Can you work these out from the model? Positions are in its coordinate system, mm. Face numbers are marked on the shaded views. A direction names the side the tool comes from. Give positions to 0.01 mm unless a question says otherwise; leave off trailing zeros. Order: outer loops, then holes, each group sorted by start corner. A loop starts at its lowest first (then second) coordinate and runs counter-clockwise, first axis right, second up. Notation, with made-up numbers: M -36.5,-12.75 L 1.5,-12.75 A23 cw 1.5,13.25 Z; hole C -3.5,86.5 d5. An arc over 180 degrees is marked long. One line per question, with ' | ' between items. Start each with the question number.
1) I'm going to push flat-ended pins straight in: pin 1 Ø2.5 at (x, z) = (255.5, 19) entering from +Y; pin 2 Ø6.5 at (x, y) = (270, -10) entering from +Z; pin 3 Ø3 at (x, y) = (206.5, -0.5) entering from +Z. Where does each tip first touch, or does it pass through?
2) For the marked faces 4 and 5, which set-ups out of +Z, -Z, +X, -X, +Y, -Y let a thin tool reach every point of the face, with its end or its side?
3) If we section it at D-D, the plane z = 14: Please give me the cut outline in (x, y).
4) If we section it at A-A, the plane z = 49: Please give me the cut outline in (x, y), plus the area to 3 significant figures.
5) Please list where these lines run through material, in increasing order: line 1 along Y through (x, z) = (10, 2.5); line 2 along X through (y, z) = (4, 20); line 3 along X through (y, z) = (17.05, 20). Write a range as [from, to].
6) Thinking about a two-plate mould opening in X: for the marked faces 1, 2 and 3, which applies, +X half, -X half, draft (parallel to the pull), parting line (faces both ways), or undercut?
7) If we section it at C-C, the plane x = 98.5: Please give me the cut outline in (y, z).
8) If we section it at B-B, the plane y = 3: Please give me the cut outline in (x, z), plus the area to 3 significant figures.
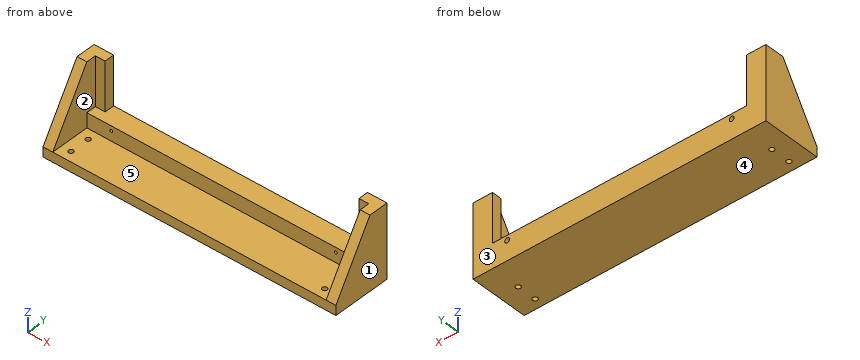
Autodesk Inventor part; units mm, degrees
ref_plane "작업 평면1" through (140, -40, 0) normal (1, 0, 0) x (0, 0, -1)
ref_plane "YZ Plane" through (0, 0, 0) normal (1, 0, 0) x (0, 1, 0)
ref_plane "XZ Plane" through (0, 0, 0) normal (0, 1, 0) x (-1, 0, 0)
sketch "스케치1" plane through (0, 0, 0) normal (0, 0, 1) x (1, 0, 0)
  line L0 (0, 10) -> (0, 0)
  line L1 (-10, 10) -> (-10, 20)
  line L2 (-10, 20) -> (290, 20)
  line L3 (290, 20) -> (290, 10)
  line L4 (0, 0) -> (280, 0)
  line L5 (290, 10) -> (290, -40)
  line L6 (-10, 10) -> (-10, -40)
  line L7 (-10, -40) -> (290, -40)
  line L8 (0, 10) -> (10, 10)
  line L9 (10, 10) -> (10, 20)
  line L10 (140, 20) -> (140, 10)
  line L11 (0, 0) -> (-10, 0)
  line L12 (280, 10) -> (280, 0)
  line L13 (280, 10) -> (270, 10)
  line L14 (270, 10) -> (270, 20)
  line L15 (280, 0) -> (290, 0)
  point P0 (140, 0)
  dimension "d2" = 10
  dimension "d5" = 10
  dimension "d6" = 300
  dimension "d9" = 60
  dimension "d12" = 10
  dimension "d13" = 10
extrude "돌출1" add sketch "스케치1" along normal blind 25 contours L8 L9 L2 L14 L13 L12 L4 L0 | L0 L11 L6 L1 L2 L9 L8 | L12 L13 L14 L2 L3 L5 L15
extrude "돌출2" add sketch "스케치1" along normal blind 10 contours L8 L9 L2 L14 L13 L12 L4 L0 | L4 L15 L5 L7 L6 L11
extrude "돌출3" add sketch "스케치1" along normal blind 75 contours L0 L11 L6 L1 L2 L9 L8 | L12 L13 L14 L2 L3 L5 L15
sketch "스케치2" plane through (-10, -40, 0) normal (-1, 0, 0) x (0, 0, 1)
  line L0 (0, 60) -> (0, 0)
  line L1 (0, 0) -> (10, 0)
  line L2 (10, 40) -> (10, 0)
  line L3 (10, 40) -> (75, 40)
  line L4 (75, 60) -> (75, 40)
  line L5 (0, 60) -> (75, 60)
  line L6 (75, 40) -> (10, 0)
  point P0 (0, 40)
extrude "돌출4" add sketch "스케치2" against normal up to surface (10 mm away) contours L2 L3 L6
ref_plane "작업 평면1" through (140, -40, 0) normal (1, 0, 0) x (0, 0, -1)
mirror "미러1" about plane through (140, -40, 0) normal (1, 0, 0) of "돌출4"
sketch "스케치3" plane through (0, 0, 10) normal (0, 0, 1) x (1, 0, 0)
  circle A0 centre (10, -10) radius 2.5
  circle A1 centre (270, -10) radius 2.5
  line L0 (270, 20) -> (10, 20)
  line L1 (290, -40) -> (290, 0)
  line L2 (-10, -40) -> (-10, 0)
  circle A2 centre (10, -30) radius 2.5
  circle A3 centre (270, -30) radius 2.5
  point P0 (0, 0)
  dimension "d18" = 30
  dimension "d19" = 5
  dimension "d20" = 20
  dimension "d21" = 20
  dimension "d24" = 5
  dimension "d25" = 20
extrude "돌출5" cut sketch "스케치3" against normal through all
sketch "스케치4" plane through (-10, 20, 0) normal (0, 1, 0) x (1, 0, 0)
  line L0 (280, -25) -> (280, -75)
  line L1 (20, -25) -> (20, -75)
  line L2 (280, -25) -> (20, -25)
  point P0 (10, 0)
  point P1 (35, -20)
  point P2 (265, -20)
  dimension "d26" = 15
  dimension "d27" = 15
  dimension "d28" = 5
hole "구멍1" at (25, 20, 20) at (255, 20, 20) direction (0, -1, 0) diameter 3 end through all counterbore diameter 5 counterbore depth 5
properties part number "ModuleConnector"
Results found:
1) pin 1: stops at y = 15 | pin 2: stops at z = 10 | pin 3: stops at z = 25
2) face 4: -Z, +X, -X, +Y, -Y | face 5: +Z, -Y
3) outline: M -10,-37.54 L 0,-37.54 L 0,0 L 280,0 L 280,-37.54 L 290,-37.54 L 290,20 L -10,20 Z
4) outline: M -10,-16 L 0,-16 L 0,10 L 10,10 L 10,20 L -10,20 Z; M 270,10 L 280,10 L 280,-16 L 290,-16 L 290,20 L 270,20 Z | area: 920 mm²
5) line 1: y = [-40, -32.5], [-27.5, -12.5], [-7.5, 20] | line 2: x = [-10, 23.5], [26.5, 253.5], [256.5, 290] | line 3: x = [-10, 22.5], [27.5, 252.5], [257.5, 290]
6) face 1: +X half | face 2: undercut | face 3: draft
7) outline: M -40,0 L 20,0 L 20,25 L 0,25 L 0,10 L -40,10 Z
8) outline: M -10,0 L 290,0 L 290,75 L 280,75 L 280,25 L 0,25 L 0,75 L -10,75 Z; hole C 25,20 d3; hole C 255,20 d3 | area: 8,490 mm²
